```python
from build123d import *

# Parameters (mm, degrees)
F1_DEPTH = 38.1
F2_R     = 9.525
F3_DEPTH = 38.101


with BuildPart() as f1:
    # F0 (on Front) → F1 (new body)
    with BuildSketch(Plane.XZ):
        Polygon((0, 63.5), (0, 0), (101.6, 0), (101.6, 25.4), (25.4, 63.5), align=None)
    extrude(amount=F1_DEPTH)

    # F2 (on face) → F3 (cut, through all)
    with BuildSketch(Plane.XZ.offset(38.1)):
        with Locations((25.4, 25.4)):
            Circle(F2_R)
    extrude(amount=-F3_DEPTH, mode=Mode.SUBTRACT)


solid = f1.part
```
Read the model definition and answer for the solid it produces. Units are mm, in the model's axes. Give positions to 0.01 mm unless a question says otherwise; leave off trailing zeros. Write each loop counter-clockwise with the first axis right and the second up, starting at its lowest first coordinate (ties: lowest second). Pieces come first, ordered by that corner, then holes. Notation, with made-up numbers: (18, -33) -> (26, -33) arc R20 cw to (26, -11) -> close; hole circle Ø1 at (17, 24). An arc over 180 degrees is marked (long way). Answer in a Markdown table with one row per item.
1) Section A-A on z = 33 is taken. Give the vertices of the cut face in (x, y).
Results list:
| item | result |
|---|---|
| outline | (0, -38.1) -> (19.66, -38.1) -> (19.66, 0) -> (0, 0) -> close; (31.14, -38.1) -> (86.4, -38.1) -> (86.4, 0) -> (31.14, 0) -> close |
2) Section C-C on x = 28.5 is taken. Give the vertices of the cut face in (y, z).
Results list:
| item | result |
|---|---|
| outline | (-38.1, 0) -> (0, 0) -> (0, 16.39) -> (-38.1, 16.39) -> close; (-38.1, 34.41) -> (0, 34.41) -> (0, 61.95) -> (-38.1, 61.95) -> close |
3) Straight lines are drawn through the part: line 1 (Z direction, x = 25.4, y = -29.5) (3 decimals); line 2 (X direction, y = -11, z = 25); line 3 (Z direction, x = 20, y = -33). For each, find the intervals that lie inside material, in ascending order. Write a range as [from, to].
Results list:
| item | result |
|---|---|
| line 1 | [0, 15.875], [34.925, 63.5] |
| line 2 | [0, 15.88], [34.92, 101.6] |
| line 3 | [0, 17.55], [33.25, 63.5] |
4) Each of these flat-tipped pins is pushed along its axis until it touches: pin 1 Ø4 at (y, z) = (-30, 48.5) entering from +X; pin 2 Ø5 at (x, y) = (91, -13.5) entering from +Z; pin 3 Ø2 at (x, y) = (71, -25) entering from +Z. Where does it stop, or does it pass through?
Results list:
| item | result |
|---|---|
| pin 1 | x = 59.4 |
| pin 2 | z = 31.95 |
| pin 3 | z = 41.2 |
5) Determine the mould class of faces 1 (the cylindrical face through (15.884, -19.317, 25.819)), 2 (the flat face through (13, -19, 63.5)), 3 (the flat face through (0, -19, 32)) for opening direction X: released by +X, released by -X, zero draft, split by the parting line, or undercut.
Results list:
| item | result |
|---|---|
| face 1 | undercut |
| face 2 | zero draft |
| face 3 | released by -X |
6) Section D-D on x = 43 is taken. Give the vertices of the cut face in (y, z), plus the area to 3 significant figures.
Results list:
| item | result |
|---|---|
| outline | (-38.1, 0) -> (0, 0) -> (0, 54.7) -> (-38.1, 54.7) -> close |
| area | 2,080 mm^2 |
7) Section B-B on y = -27 is taken. Give the vertices of the cut face in (x, z) (3 decimals).
Results list:
| item | result |
|---|---|
| outline | (0, 0) -> (101.6, 0) -> (101.6, 25.4) -> (25.4, 63.5) -> (0, 63.5) -> close; hole circle Ø19.05 at (25.4, 25.4) |
